The figure shows three views and two pictorial views of one solid part (mm, origin at its lowest corner). Answer the questions. Coordinates: 2 decimals unless noted, no trailing zeros. Loops run counter-clockwise (first coordinate to the right, second up) from the corner with the lowest first, then second, coordinate; pieces in that order, holes last. Notation, with made-up numbers: M 38,84.25 L 92,84.25 A17 cw 92,97.25 Z; hole C 22,83.5 d3. An arc over 180 degrees is marked long. Answer as a JSON object with one key per item and string values. Group by question number.
1. A cutting plane is placed at C-C on x = 7.5. Give the vertices of the cut face in (y, z), and give its area (3 significant figures).
2. A cutting plane is placed at A-A on x = 20. Give the vertices of the cut face in (y, z).
3. Straight lines are drawn through the part: L1, parallel to Y at x = 7.5, z = 0.8; L2, parallel to Y at x = 20, z = 1.6; L3, parallel to Y at x = 18, z = 1.2. For each, find the intervals that lie inside material, in ascending order.
4. Given pin 1 (12 mm diameter, centred on x = 26, y = 16.5, fed in from +Z); pin 2 (1 mm diameter, centred on x = 22, z = 1.5, fed in from +Y), each flat-ended and moving along its own axis, determine where each tip first touches the part or whether it passes through.
5. A cutting plane is placed at D-D on z = 0.55. Give the vertices of the cut face in (x, y), and give its area (3 significant figures).
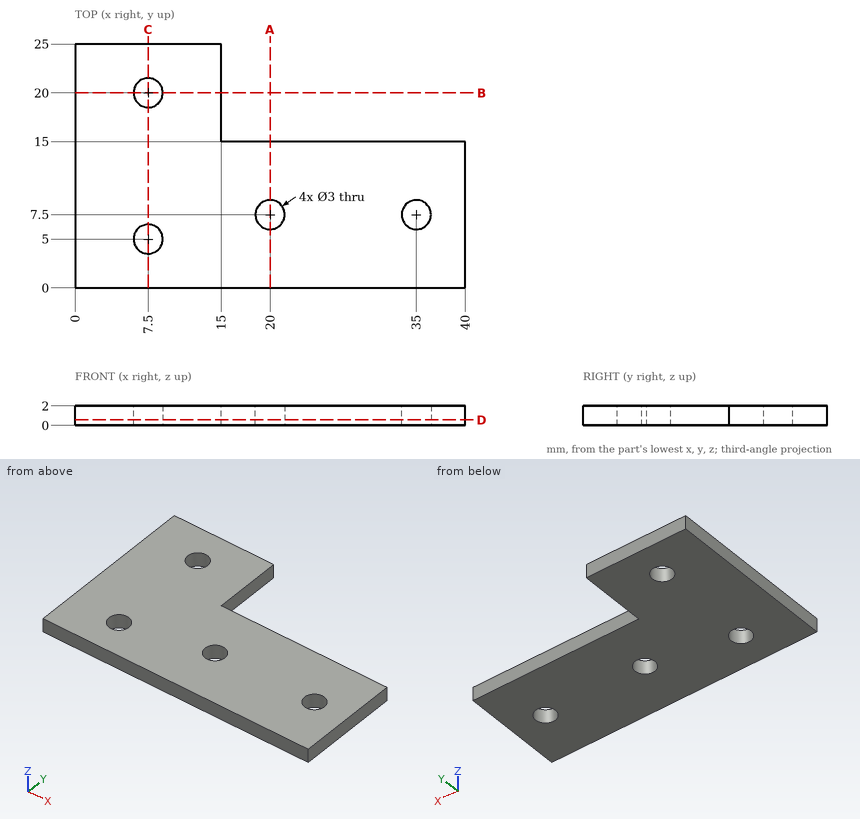
From the geometry:
{
 "1": {"outline": "M 0,0 L 3.5,0 L 3.5,2 L 0,2 Z; M 6.5,0 L 18.5,0 L 18.5,2 L 6.5,2 Z; M 21.5,0 L 25,0 L 25,2 L 21.5,2 Z", "area": "38.0 mm²"},
 "2": {"outline": "M 0,0 L 6,0 L 6,2 L 0,2 Z; M 9,0 L 15,0 L 15,2 L 9,2 Z"},
 "3": {"L1": "y = 0 to 3.5, 6.5 to 18.5, 21.5 to 25", "L2": "y = 0 to 6, 9 to 15", "L3": "y = 0 to 15"},
 "4": {"pin 1": "stops at z = 2", "pin 2": "stops at y = 15"},
 "5": {"outline": "M 0,0 L 40,0 L 40,15 L 15,15 L 15,25 L 0,25 Z; hole C 7.5,5 d3; hole C 7.5,20 d3; hole C 20,7.5 d3; hole C 35,7.5 d3", "area": "722 mm²"}
}
